Autodesk Inventor part; units mm, degrees
ref_plane "YZ Plane" through (0, 0, 0) normal (1, 0, 0) x (0, 1, 0)
ref_plane "XZ Plane" through (0, 0, 0) normal (0, 1, 0) x (-1, 0, 0)
ref_plane "XY Plane" through (0, 0, 0) normal (0, 0, 1) x (1, 0, 0)
sketch "Boceto2" plane through (0, 0, 0) normal (0, 1, 0) x (-1, 0, 0)
  line L0 (0, 0) -> (-17, 0)
  line L1 (-17, 0) -> (-17, -21)
  line L2 (-17, -21) -> (0, -21)
  line L3 (0, -21) -> (0, 0)
  dimension "d0" = 17
  dimension "d1" = 21
  dimension "d2" = 17
extrude "Extrusión1" add sketch "Boceto2" along normal blind 2
sketch "Boceto3" plane through (0, 2, 0) normal (0, 1, 0) x (1, 0, 0)
  line L0 (0, 0) -> (17, 0)
  line L1 (0, 0) -> (0, 21)
  line L2 (0, 21) -> (0, 0)
  line L3 (0, 21) -> (17, 21)
  line L4 (17, 0) -> (17, 21)
  line L5 (0, 0) -> (17, 0)
  line L6 (17, 0) -> (17, 21)
  dimension "d5" = 21
extrude "Extrusión3" add sketch "Boceto3" along normal blind 19
sketch "Boceto5" plane through (0, 21, 0) normal (0, 1, 0) x (1, 0, 0)
  line L0 (17, 21) -> (0, 21)
  line L1 (2, 21) -> (2, 2)
  line L2 (2, 2) -> (15, 2)
  line L3 (15, 2) -> (15, 21)
  line L4 (15, 21) -> (2, 21)
  point P0 (0, 0)
extrude "Extrusión5" cut sketch "Boceto5" against normal blind 19
sketch "Boceto6" plane through (17, 0, 0) normal (1, 0, 0) x (0, 0, -1)
  line L0 (0, 0) -> (21, 0)
  line L1 (0, 21) -> (21, 21)
  line L2 (21, 2) -> (0, 21)
  line L3 (0, 21) -> (21, 21)
  line L4 (21, 21) -> (21, 2)
extrude "Extrusión6" cut sketch "Boceto6" against normal blind 19
sketch "Boceto7" plane through (0, 2, 0) normal (0, 1, 0) x (1, 0, 0)
  line L0 (0, 0) -> (17, 0)
  circle A0 centre (8.5, 16) radius 3
extrude "Extrusión7" cut sketch "Boceto7" against normal blind 19
sketch "Boceto8" plane through (15, 2, -2) normal (0, 0, -1) x (-1, 0, 0)
  line L0 (-2, -2) -> (15, -2)
  circle A0 centre (6.5, 12) radius 3
extrude "Extrusión8" cut sketch "Boceto8" against normal blind 19
properties part number "Triangulo"
Here's how the part is built. I have some questions about the finished solid (model axes, mm). A direction names the side the tool comes from. Coordinates: 2 decimals unless noted, no trailing zeros. Order: outer loops, then holes, each group sorted by start corner. A loop starts at its lowest first (then second) coordinate and runs counter-clockwise, first axis right, second up. Notation, with made-up numbers: (52.25, 46.5) - (84.25, 46.5) arc R24 ccw to (84.25, 74.5) - close; hole circle Ø2 at (48, 13). An arc over 180 degrees is marked (long way). Use CSV: the item, a comma, the result in double quotes. Start each with the question number.
1. Suppose I cut it at A-A on x = 8.5. List the corners of the cut face in (y, z) for me, then the cut area to 3 significant figures.
2. Please list where these lines run through material, in increasing order: line 1 (Z direction, x = 8.5, y = 1.1); line 2 (X direction, y = 6.25, z = -16); line 3 (X direction, y = 1.2, z = -16). Write a range as from..to.
3. I'm going to push flat-ended pins straight in: pin 1 (8 mm diameter, centred on x = 8.5, z = -8.5, fed in from +Y); pin 2 (9.5 mm diameter, centred on x = 8.5, y = 14, fed in from -Z); pin 3 (6 mm diameter, centred on x = 3.5, z = -19, fed in from +Y). Where does each tip first touch, or does it pass through?
4. Suppose I cut it at D-D on z = -5.25. List the corners of the cut face in (x, y) for me.
5. For faces 1 (the face through (8, 2, -12)), 2 (the face through (9.15, 11.07, -1.01)), which set-ups out of +Z, -Z, +X, -X, +Y, -Y let a thin tool reach every point of the face, with its end or its side?
6. If we mould it in two halves opening along Z, with no side actions, what happens to faces 3 (the face through (0, 8, -8)), 4 (the face through (9, 1, -21)), 5 (the face through (9.884, 1.014, -13.338))? For each: +Z half, -Z half, draft (parallel to the pull), parting line (faces both ways), or undercut.
7. Suppose I cut it at B-B on y = 11.5. List the corners of the cut face in (x, z) for me.
8. Suppose I cut it at C-C on z = -15. List the corners of the cut face in (x, y) for me.
Output:
1,outline,"(0, -21) - (2, -21) - (2, -19) - (0, -19) - close; (0, -13) - (2, -13) - (2, -2) - (11, -2) - (11, 0) - (0, 0) - close; (17, -2) - (19.19, -2) - (21, 0) - (17, 0) - close"
1,area,"54.2 mm2"
2,line 1,"z = -21..-19, -13..0"
2,line 2,"x = 0..2, 15..17"
2,line 3,"x = 0..5.5, 11.5..17"
3,pin 1,"stops at y = 2"
3,pin 2,"stops at z = -2"
3,pin 3,"stops at y = 6.16"
4,outline,"(0, 0) - (17, 0) - (17, 16.25) - (15, 16.25) - (15, 2) - (2, 2) - (2, 16.25) - (0, 16.25) - close"
5,face 1,"-Z, +Y"
5,face 2,"+Z, -Z"
6,face 3,"draft"
6,face 4,"-Z half"
6,face 5,"undercut"
7,outline,"(0, -10.5) - (2, -10.5) - (2, -2) - (6.84, -2) - (6.84, 0) - (0, 0) - close; (10.16, -2) - (15, -2) - (15, -10.5) - (17, -10.5) - (17, 0) - (10.16, 0) - close"
8,outline,"(0, 0) - (5.67, 0) - (5.67, 2) - (2, 2) - (2, 7.43) - (0, 7.43) - close; (11.33, 0) - (17, 0) - (17, 7.43) - (15, 7.43) - (15, 2) - (11.33, 2) - close"
